Part print with two shaded views. Sizes in mm from the minimum x, y, z corner. Round coordinates to 2 decimals unless told otherwise and drop trailing zeros. Loops run counter-clockwise (first coordinate to the right, second up) from the corner with the lowest first, then second, coordinate; pieces in that order, holes last. Notation, with made-up numbers: (-17.5, 67.25) - (-13.5, 67.25) arc R18 cw to (-13.5, 85.25) - close; hole circle Ø3 at (3.5, -19). An arc over 180 degrees is marked (long way). One line per question, with ' | ' between items.
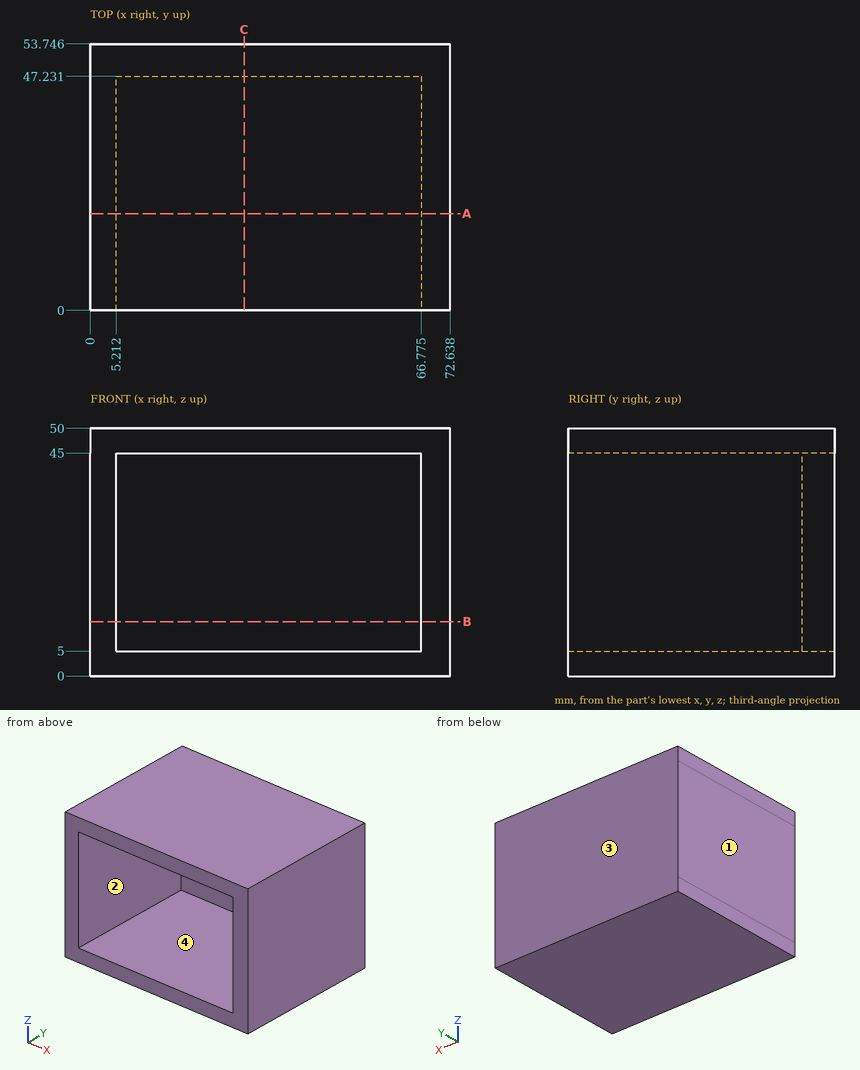
(1) Cut at A-A, the plane y = 19.5. Write the cut outline in (x, z) (1 decimal).
Results found:
outline: (0, 0) - (72.6, 0) - (72.6, 50) - (0, 50) - close; hole (5.2, 5) - (66.8, 5) - (66.8, 45) - (5.2, 45) - close
(2) Cut at C-C, the plane x = 31. Write the cut outline in (y, z), then the cut area to 3 significant figures.
Results found:
outline: (0, 0) - (53.75, 0) - (53.75, 50) - (0, 50) - (0, 45) - (47.23, 45) - (47.23, 5) - (0, 5) - close | area: 798 mm²
(3) Cut at B-B, the plane z = 11. Write the cut outline in (x, y) (1 decimal).
Results found:
outline: (0, 0) - (5.2, 0) - (5.2, 47.2) - (66.8, 47.2) - (66.8, 0) - (72.6, 0) - (72.6, 53.7) - (0, 53.7) - close
(4) Two-plate mould, pull along X, no slides. Class the marked faces 1, 2, 3 and 4: released by +X, released by -X, zero draft, split by the parting line, or undercut.
Results found:
face 1: released by -X | face 2: undercut | face 3: zero draft | face 4: undercut
(5) Probe L1, parallel to X at y = 39, z = 19 (1 decimal); L2, parallel to Z at x = 14.5, y = 38; L3, parallel to Y at x = 34.5, z = 12.5. List the from-to ranges inside material, lowest first.
Results found:
L1: x = 0 to 5.2, 66.8 to 72.6 | L2: z = 0 to 5, 45 to 50 | L3: y = 47.23 to 53.75
